```python
from build123d import *

# Parameters (mm, degrees)
SKETCH1_W           = 5.7
SKETCH1_H           = 8.509
SKETCH1_R           = 1.778
SKETCH1_R_2         = 1.8288
BOSS_EXTRUDE1_DEPTH = 6


with BuildPart() as part:
    # Sketch1 → Boss-Extrude1 (new body)
    with BuildSketch(Plane(origin=(0, 0, 0), x_dir=(1, 0, 0), z_dir=(0, 1, 0))):
        with BuildLine():
            ThreePointArc((-203.2, -19.05), (-199.480256121, -28.030256121), (-190.5, -31.75))
            Line((-190.5, -31.75), (190.5, -31.75))
            ThreePointArc((190.5, -31.75), (199.480256121, -28.030256121), (203.2, -19.05))
            Line((203.2, -19.05), (203.2, 19.05))
            ThreePointArc((203.2, 19.05), (199.480256121, 28.030256121), (190.5, 31.75))
            Line((190.5, 31.75), (178.816, 31.75))
            Line((178.816, 31.75), (178.816, 26.035))
            Line((178.816, 26.035), (178.816, 17.526))
            Line((178.816, 17.526), (173.116, 17.526))
            Line((173.116, 17.526), (173.116, 26.035))
            Line((173.116, 26.035), (173.116, 31.75))
            Line((173.116, 31.75), (25.4, 31.75))
            ThreePointArc((25.4, 31.75), (16.419743879, 28.030256121), (12.7, 19.05))
            Line((12.7, 19.05), (12.7, 0))
            ThreePointArc((12.7, 0), (0, -12.7), (-12.7, 0))
            Line((-12.7, 0), (-12.7, 19.05))
            ThreePointArc((-12.7, 19.05), (-16.419743879, 28.030256121), (-25.4, 31.75))
            Line((-25.4, 31.75), (-173.116, 31.75))
            Line((-173.116, 31.75), (-173.116, 26.035))
            Line((-173.116, 26.035), (-173.116, 17.526))
            Line((-173.116, 17.526), (-178.816, 17.526))
            Line((-178.816, 17.526), (-178.816, 26.035))
            Line((-178.816, 26.035), (-178.816, 31.75))
            Line((-178.816, 31.75), (-190.5, 31.75))
            ThreePointArc((-190.5, 31.75), (-199.480256121, 28.030256121), (-203.2, 19.05))
            Line((-203.2, 19.05), (-203.2, -19.05))
        make_face()
        with Locations((-175.966, -21.3995)):
            Rectangle(SKETCH1_W, SKETCH1_H, mode=Mode.SUBTRACT)
        with Locations(Location((-175.966, -10.6045, 0), (0, 0, 270))):
            Circle(SKETCH1_R, mode=Mode.SUBTRACT)
        with Locations((175.966, -21.3995)):
            Rectangle(SKETCH1_W, SKETCH1_H, mode=Mode.SUBTRACT)
        with Locations(Location((175.966, -10.6045, 0), (0, 0, 270))):
            Circle(SKETCH1_R, mode=Mode.SUBTRACT)
        with Locations((-175.966, 0.1905)):
            Rectangle(SKETCH1_W, SKETCH1_H, mode=Mode.SUBTRACT)
        with Locations(Location((-175.966, 10.9855, 0), (0, 0, 270))):
            Circle(SKETCH1_R, mode=Mode.SUBTRACT)
        with Locations(Location((-65.5, 12.7, 0), (0, 0, 270))):
            Circle(SKETCH1_R_2, mode=Mode.SUBTRACT)
        with Locations(Location((65.5, 12.7, 0), (0, 0, 270))):
            Circle(SKETCH1_R_2, mode=Mode.SUBTRACT)
        with Locations((175.966, 0.1905)):
            Rectangle(SKETCH1_W, SKETCH1_H, mode=Mode.SUBTRACT)
        with Locations(Location((175.966, 10.9855, 0), (0, 0, 270))):
            Circle(SKETCH1_R, mode=Mode.SUBTRACT)
    extrude(amount=BOSS_EXTRUDE1_DEPTH)


solid = part.part
```
Could you check a few things on this model? Use its own coordinates, in mm. A direction names the side the tool comes from. Round coordinates to 2 decimals unless told otherwise and drop trailing zeros. Loops run counter-clockwise (first coordinate to the right, second up) from the corner with the lowest first, then second, coordinate; pieces in that order, holes last. Notation, with made-up numbers: (18.25, -36) - (59.25, -36) arc R21 cw to (59.25, -23) - close; hole circle Ø4 at (28, -30.5). An arc over 180 degrees is marked (long way). Answer as CSV lines item,"result".
1. We'd pull the mould along X, two halves only. Please class faces 1 (the face through (199.38, 2.96, 28.13)), 2 (the face through (-199.38, 2.96, -28.13)), 3 (the face through (0.279, 2.958, 12.697)): +X half, -X half, draft (parallel to the pull), parting line (faces both ways), or undercut.
Filled in:
face 1,"+X half"
face 2,"-X half"
face 3,"undercut"
2. On a 3-axis mill with a long thin cutter (end or side, diameter ignored), from which of +Z, -Z, +X, -X, +Y, -Y can I reach the whole of each face in a straight line? I mean faces 4 (the face through (-16.32, 2.96, -27.93)), 5 (the face through (-3, 6, 14)). Say none if no direction works.
Filled in:
face 4,"-Z, +Y, -Y"
face 5,"+Z, -Z, +X, -X, +Y"
3. Please list where these lines run through material, in increasing order: line 1 along X through (y, z) = (4.15, 18); line 2 along X through (y, z) = (4.5, -4); line 3 along X through (y, z) = (2.2, -7). Write a range as [from, to].
Filled in:
line 1,"x = [-203.2, -178.82], [-173.12, 173.12], [178.82, 203.2]"
line 2,"x = [-203.2, -178.82], [-173.12, -12.7], [12.7, 173.12], [178.82, 203.2]"
line 3,"x = [-203.2, -12.7], [12.7, 203.2]"
4. For pin 1 Ø3 at (y, z) = (2, -21.5) entering from +X; pin 2 Ø3 at (y, z) = (4, -26) entering from -X; pin 3 Ø3 at (x, y) = (176, 1.5) entering from -Z, each with a flat end and sliding along its axis, tell me the tip position at first contact or that it passes through.
Filled in:
pin 1,"stops at x = 203.16"
pin 2,"stops at x = -201.97"
pin 3,"stops at z = -17.53"
5. I want a section at B-B on y = 2.4. Count the separate pieces of the cut face and the enclosed holes in it, then the cut area to 3 significant figures.
Filled in:
separate pieces,"1"
enclosed holes,"10"
area,"24,100 mm^2"
6. I want a section at A-A on x = 0. List the corners of the cut face in (y, z) for me, then the cut area to 3 significant figures.
Filled in:
outline,"(0, 12.7) - (6, 12.7) - (6, 31.75) - (0, 31.75) - close"
area,"114 mm^2"
